```python
from build123d import *

# Parameters (mm, degrees)
SKETCH1_R           = 35.5
BOSS_EXTRUDE1_DEPTH = 1.5
SKETCH2_R           = 26
BOSS_EXTRUDE2_DEPTH = 1
SKETCH3_R           = 25
BOSS_EXTRUDE3_DEPTH = 19
SKETCH4_R           = 12
CUT_EXTRUDE1_DEPTH  = 56.222278113
SKETCH5_R           = 7.5
CUT_EXTRUDE2_DEPTH  = 56.222278113
FILLET1_R           = 1
SKETCH6_R           = 30.018937713
SKETCH6_R_2         = 20
CUT_EXTRUDE3_DEPTH  = 12
CHAMFER2_SIZE       = 2.5
BOSS_EXTRUDE4_START = 8
SKETCH8_R           = 25
BOSS_EXTRUDE4_DEPTH = 8
SKETCH10_R          = 7.5
CUT_EXTRUDE6_DEPTH  = 60.004237189
SKETCH7_R           = 1.75
CUT_EXTRUDE4_DEPTH  = 60.004237136
BOSS_EXTRUDE5_START = 1
SKETCH11_R          = 26
SKETCH11_R_2        = 25
BOSS_EXTRUDE5_DEPTH = 1
SKETCH9_R           = 12
CUT_EXTRUDE5_DEPTH  = 60.004237189
CHAMFER1_SIZE       = 1


with BuildPart() as part:
    # Sketch1 → Boss-Extrude1 (new, symmetric)
    with BuildSketch(Plane(origin=(0, 0, 0), x_dir=(1, 0, 0), z_dir=(0, 1, 0))):
        with Locations(Location((0, 0, 0), (0, 0, 270))):
            Circle(SKETCH1_R)
    extrude(amount=BOSS_EXTRUDE1_DEPTH, both=True)

    # Sketch2 → Boss-Extrude2 (add)
    with BuildSketch(Plane(origin=(0, 1.5, 0), x_dir=(1, 0, 0), z_dir=(0, 1, 0))):
        with Locations(Location((0, 0, 0), (0, 0, 270))):
            Circle(SKETCH2_R)
    extrude(amount=BOSS_EXTRUDE2_DEPTH)

    # Sketch3 → Boss-Extrude3 (add)
    with BuildSketch(Plane(origin=(0, 2.5, 0), x_dir=(1, 0, 0), z_dir=(0, 1, 0))):
        with Locations(Location((0, 0, 0), (0, 0, 270))):
            Circle(SKETCH3_R)
    extrude(amount=BOSS_EXTRUDE3_DEPTH)

    # Sketch4 → Cut-Extrude1 (cut, through all)
    with BuildSketch(Plane(origin=(0, 21.5, 0), x_dir=(1, 0, 0), z_dir=(0, 1, 0))):
        with Locations(Location((0, 15.5, 0), (0, 0, 270))):
            Circle(SKETCH4_R)
        with Locations(Location((13.423393759, -7.75, 0), (0, 0, 270))):
            Circle(SKETCH4_R)
        with Locations(Location((-13.423393759, -7.75, 0), (0, 0, 270))):
            Circle(SKETCH4_R)
    extrude(amount=-CUT_EXTRUDE1_DEPTH, mode=Mode.SUBTRACT)

    # Sketch5 → Cut-Extrude2 (cut, through all)
    with BuildSketch(Plane(origin=(0, 21.5, 0), x_dir=(1, 0, 0), z_dir=(0, 1, 0))):
        Circle(SKETCH5_R)
    extrude(amount=-CUT_EXTRUDE2_DEPTH, mode=Mode.SUBTRACT)

    # Fillet1
    fillet1_edges = [part.edges().sort_by_distance(p)[0] for p in [
        (-24.723095296, 12, 3.710600891),
        (-15.575022283, 12, 19.555528141),
        (15.575022283, 12, 19.555528141),
        (24.723095296, 12, 3.710600891),
        (9.148073013, 12, -23.266129032),
        (-9.148073013, 12, -23.266129032),
    ]]
    fillet(fillet1_edges, radius=FILLET1_R)

    # Sketch6 → Cut-Extrude3 (cut)
    with BuildSketch(Plane(origin=(0, 21.5, 0), x_dir=(1, 0, 0), z_dir=(0, 1, 0))):
        Circle(SKETCH6_R)
        Circle(SKETCH6_R_2, mode=Mode.SUBTRACT)
    extrude(amount=-CUT_EXTRUDE3_DEPTH, mode=Mode.SUBTRACT)

    # Chamfer2
    chamfer2_edges = [part.edges().sort_by_distance(p)[0] for p in [
        (17.320508076, 9.5, -10),
        (-17.320508076, 9.5, -10),
        (0, 9.5, 20),
    ]]
    chamfer(chamfer2_edges, length=CHAMFER2_SIZE)

    # Sketch8 → Boss-Extrude4 (add)
    with BuildSketch(Plane.XZ.offset(1.5).offset(BOSS_EXTRUDE4_START)):
        with Locations(Location((0, 0, 0), (0, 0, 51.464391847))):
            Circle(SKETCH8_R)
    extrude(amount=-BOSS_EXTRUDE4_DEPTH)

    # Sketch10 → Cut-Extrude6 (cut, through all)
    with BuildSketch(Plane.XZ.offset(9.5)):
        with Locations(Location((0, 0, 0), (0, 0, 79.011010973))):
            Circle(SKETCH10_R)
    extrude(amount=-CUT_EXTRUDE6_DEPTH, mode=Mode.SUBTRACT)

    # Sketch7 → Cut-Extrude4 (cut, through all)
    with BuildSketch(Plane(origin=(0, 21.5, 0), x_dir=(1, 0, 0), z_dir=(0, 1, 0))):
        with Locations(Location((0, -15, 0), (0, 0, 270))):
            Circle(SKETCH7_R)
        with Locations(Location((-12.990381057, 7.5, 0), (0, 0, 270))):
            Circle(SKETCH7_R)
        with Locations(Location((12.990381057, 7.5, 0), (0, 0, 270))):
            Circle(SKETCH7_R)
    extrude(amount=-CUT_EXTRUDE4_DEPTH, mode=Mode.SUBTRACT)

    # Sketch11 → Boss-Extrude5 (add)
    with BuildSketch(Plane.XZ.offset(1.5).offset(BOSS_EXTRUDE5_START)):
        with Locations(Location((0, 0, 0), (0, 0, 46.639268068))):
            Circle(SKETCH11_R)
        with Locations(Location((0, 0, 0), (0, 0, 270))):
            Circle(SKETCH11_R_2, mode=Mode.SUBTRACT)
    extrude(amount=-BOSS_EXTRUDE5_DEPTH)

    # Sketch9 → Cut-Extrude5 (cut, through all)
    with BuildSketch(Plane.XZ.offset(9.5)):
        with Locations((-13.423393759, 7.75)):
            Circle(SKETCH9_R)
        with Locations((13.423393759, 7.75)):
            Circle(SKETCH9_R)
        with Locations((0, -15.5)):
            Circle(SKETCH9_R)
    extrude(amount=-CUT_EXTRUDE5_DEPTH, mode=Mode.SUBTRACT)

    # Chamfer1
    chamfer1_2_edges = [part.edges().sort_by_distance(p)[0] for p in [
        (-22.516660498, 1.5, -13),
        (22.516660498, 1.5, -13),
        (0, 1.5, 26),
        (22.516660498, -1.5, -13),
        (0, -1.5, 26),
        (-22.516660498, -1.5, -13),
    ]]
    chamfer(chamfer1_2_edges, length=CHAMFER1_SIZE - 0.0001)  # a hair under: the kernel refuses the full size


solid = part.part
```
Design review of the part built by this model. Coordinates are the model's own, in mm. A direction names the side the tool comes from. Coordinates: 2 decimals unless noted, no trailing zeros. Order: outer loops, then holes, each group sorted by start corner. A loop starts at its lowest first (then second) coordinate and runs counter-clockwise, first axis right, second up. Notation, with made-up numbers: M 27.25,-18.75 L 34.25,-18.75 A14 ccw 34.25,5.25 Z; hole C -23.75,29.5 d7. An arc over 180 degrees is marked long. Answer as a JSON object with one key per item and string values. Group by question number.
1) Add section C-C, the plane z = 15. Write out the cut boundary in (x, y).
2) Add section A-A, the plane x = 0. Count the separate pieces of the cut face and the enclosed holes in it, then the cut area to 3 significant figures.
3) Mouldability with a two-part tool opening along Z and no side actions: class faces 1 (the cylindrical face through (-6.505, 5.783, -3.733)), 2 (the cylindrical face through (0, 17, 20)), 3 (the flat face through (-17, -9.5, -9)) as pulls with the +Z half, pulls with the -Z half, needs draft (parallel to the pull), parting line crosses it, or undercut.
4) Tool access review of faces 4 (the flat face through (0, 9.5, 23)), 5 (the cylindrical face through (0, -6, 25)), 6 (the cylindrical face through (-17.264, 16.816, -10.098)), 7 (the flat face through (-24, 1.5, -13)), 8 (the cylindrical face through (6.485, 5.783, -3.767)): name each direction out of +Z, -Z, +X, -X, +Y, -Y from which nothing blocks a thin tool from reaching the whole face with its end or side.
5) For pin 1 (10 mm diameter, centred on y = -1.5, z = 14, fed in from +X); pin 2 (5.5 mm diameter, centred on x = -3.5, z = 23.5, fed in from +Y); pin 3 (4 mm diameter, centred on y = 5.5, z = 23, fed in from -X), all flat-tipped, find the tip position at first contact; note any pin that passes through.
6) Add section B-B, the plane y = 14. Write out the cut boundary in (x, z), then the cut area to 3 significant figures.
7) Wall thickness on L1, parallel to X at y = 11.5, z = 7.75; L2, parallel to X at y = 15, z = -7.5; L3, parallel to X at y = 7, z = -6: over which ranges is each line inside the solid? List them lowest first.
Computed values:
{
 "1": {"outline": "M -32.18,-1.5 L -22.99,-1.5 L -22.99,1.5 L -32.18,1.5 Z; M -3.86,-9.5 L -1.75,-9.5 L -1.75,21.5 L -3.86,21.5 Z; M 1.75,-9.5 L 3.86,-9.5 L 3.86,21.5 L 1.75,21.5 Z; M 22.99,-1.5 L 32.18,-1.5 L 32.18,1.5 L 22.99,1.5 Z"},
 "2": {"separate pieces": "3", "enclosed holes": "0", "area": "436 mm^2"},
 "3": {"face 1": "undercut", "face 2": "pulls with the +Z half", "face 3": "needs draft"},
 "4": {"face 4": "+Z, +Y", "face 5": "+Z, -Y", "face 6": "-Z, -X, +Y", "face 7": "+Y", "face 8": "+Y, -Y"},
 "5": {"pin 1": "stops at x = 34.34", "pin 2": "stops at y = 10.99", "pin 3": "stops at x = -13.11"},
 "6": {"outline": "M -19.86,-2.38 A20 ccw -11.99,-16.01 A12 cw -5.66,-4.92 A7.5 cw -7.09,-2.44 A12 cw Z; M -7.87,18.39 A12 cw -1.43,7.36 A7.5 cw 1.43,7.36 A12 cw 7.87,18.39 A20 ccw Z; M 5.66,-4.92 A12 cw 11.99,-16.01 A20 ccw 19.86,-2.38 A12 cw 7.09,-2.44 A7.5 cw Z; hole C -12.99,-7.5 d3.5; hole C 0,15 d3.5; hole C 12.99,-7.5 d3.5", "area": "234 mm^2"},
 "7": {"L1": "x = -1.42 to 1.42", "L2": "x = -18.54 to -14.74, -11.24 to -8.94, 8.94 to 11.24, 14.74 to 18.54", "L3": "x = -24.27 to -13.89, -12.09 to -7.33, 7.33 to 12.09, 13.89 to 24.27"}
}
